```python
from build123d import *

# Parameters (mm, degrees)
BOSS_EXTRUDE1_DEPTH = 3.175
SHELL1_START        = -3.175
SHELL1_DEPTH        = 3.175
FILLET1_R           = 10.16
BOSS_EXTRUDE2_DEPTH = 3.175
SKETCH1_R           = 2.75
CUT_EXTRUDE1_DEPTH  = 81.407776093
EXTRUDE_THIN1_START = 25.4
SKETCH5_R           = 4.782
SKETCH5_R_2         = 2.75
EXTRUDE_THIN1_DEPTH = 25.4
SKETCH6_R           = 2.749999961
CUT_EXTRUDE2_DEPTH  = 85.264404295


# Read off the part's stored shape, not the designer's step: Shell1
with BuildPart() as part:
    # Sketch2 → Boss-Extrude1 (new body)
    with BuildSketch(Plane(origin=(0, 0, 0), x_dir=(1, 0, 0), z_dir=(0, 1, 0))):
        with BuildLine():
            Line((-60.494192364, -19.59062768), (-46.524192364, 43.90937232))
            ThreePointArc((-46.524192364, 43.90937232), (-42.81709678, 48.384476595), (-37.020836887, 47.969160828))
            Line((-37.020836887, 47.969160828), (50.609163113, -5.370839172))
            ThreePointArc((50.609163113, -5.370839172), (53.499476113, -12.202811), (47.939348616, -17.113486158))
            Line((47.939348616, -17.113486158), (-53.660651384, -27.273486158))
            ThreePointArc((-53.660651384, -27.273486158), (-59.037220059, -25.175205156), (-60.494192364, -19.59062768))
        make_face()
    extrude(amount=-BOSS_EXTRUDE1_DEPTH)

    # Shell1 outline → Shell1 (cut)
    with BuildSketch(Plane(origin=(0, 0, 0), x_dir=(1, 0, 0), z_dir=(0, 1, 0)).offset(SHELL1_START)):
        Polygon((-54.2925, -20.955), (47.3075, -10.795), (-40.3225, 42.545), align=None)
    extrude(amount=SHELL1_DEPTH, mode=Mode.SUBTRACT)

    # Fillet1
    fillet1_edges = [part.edges().sort_by_distance(p)[0] for p in [
        (-40.3225, -1.5875, -42.545),
        (47.3075, -1.5875, 10.795),
        (-54.2925, -1.5875, 20.955),
    ]]
    fillet(fillet1_edges, radius=FILLET1_R)

    # Sketch3 → Boss-Extrude2 (add)
    with BuildSketch(Plane(origin=(0, 0, 0), x_dir=(1, 0, 0), z_dir=(0, 1, 0))):
        with BuildLine():
            Line((-60.6425, -20.955), (-60.6425, -52.705))
            Line((-60.6425, -52.705), (53.6575, -52.705))
            Line((53.6575, -52.705), (53.6575, -10.795))
            ThreePointArc((53.6575, -10.795), (52.015723588, -15.055883787), (47.939348616, -17.113486158))
            Line((47.939348616, -17.113486158), (-53.660651384, -27.273486158))
            ThreePointArc((-53.660651384, -27.273486158), (-58.553383787, -25.663223588), (-60.6425, -20.955))
        make_face()
    extrude(amount=-BOSS_EXTRUDE2_DEPTH)

    # Sketch1 → Cut-Extrude1 (cut, through all)
    with BuildSketch(Plane(origin=(0, 0, 0), x_dir=(1, 0, 0), z_dir=(0, 1, 0))):
        with Locations(Location((-54.2925, -20.955, 0), (0, 0, 270))):
            Circle(SKETCH1_R)
        with Locations(Location((47.3075, -10.795, 0), (0, 0, 270))):
            Circle(SKETCH1_R)
        with Locations(Location((-40.3225, 42.545, 0), (0, 0, 270))):
            Circle(SKETCH1_R)
    extrude(amount=-CUT_EXTRUDE1_DEPTH, mode=Mode.SUBTRACT)

    # Sketch5 → Extrude-Thin1 (add)
    # profile 1 of 3: a face of its own
    with BuildSketch(Plane(origin=(0, 0, 0), x_dir=(1, 0, 0), z_dir=(0, 1, 0)).offset(EXTRUDE_THIN1_START)):
        with Locations((47.3075, -10.795)):
            Circle(SKETCH5_R)
        with Locations((47.3075, -10.795)):
            Circle(SKETCH5_R_2, mode=Mode.SUBTRACT)
    # profile 2 of 3: a face of its own
    with BuildSketch(Plane(origin=(0, 0, 0), x_dir=(1, 0, 0), z_dir=(0, 1, 0)).offset(EXTRUDE_THIN1_START)):
        with Locations((-54.2925, -20.955)):
            Circle(SKETCH5_R)
        with Locations((-54.2925, -20.955)):
            Circle(SKETCH5_R_2, mode=Mode.SUBTRACT)
    # profile 3 of 3: a face of its own
    with BuildSketch(Plane(origin=(0, 0, 0), x_dir=(1, 0, 0), z_dir=(0, 1, 0)).offset(EXTRUDE_THIN1_START)):
        with Locations((-40.3225, 42.545)):
            Circle(SKETCH5_R)
        with Locations((-40.3225, 42.545)):
            Circle(SKETCH5_R_2, mode=Mode.SUBTRACT)
    extrude(amount=-EXTRUDE_THIN1_DEPTH)

    # Sketch6 → Cut-Extrude2 (cut, through all)
    with BuildSketch(Plane(origin=(0, 0, 0), x_dir=(1, 0, 0), z_dir=(0, 1, 0))):
        with Locations(Location((-13.492499939, -42.705, 0), (0, 0, 270))):
            Circle(SKETCH6_R)
        with Locations(Location((6.507499939, -42.705, 0), (0, 0, 270))):
            Circle(SKETCH6_R)
    extrude(amount=-CUT_EXTRUDE2_DEPTH, mode=Mode.SUBTRACT)


solid = part.part
```
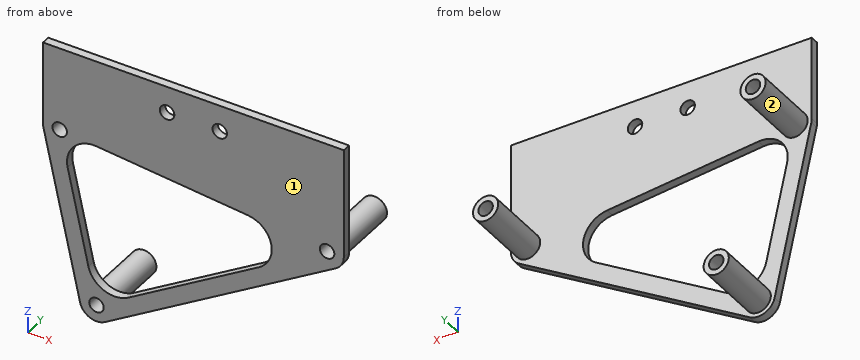
CAD build for the part. Positions are in the model's coordinates, mm. Face numbers are marked on the shaded views. A direction names the side the tool comes from. Give positions to 0.01 mm unless a question says otherwise; leave off trailing zeros. Write each loop counter-clockwise with the first axis right and the second up, starting at its lowest first coordinate (ties: lowest second). Pieces come first, ordered by that corner, then holes. Notation, with made-up numbers: M 80.25,9.25 L 99.25,9.25 A12 ccw 99.25,25.25 Z; hole C 29,52 d7. An arc over 180 degrees is marked long. Return JSON: item names as keys, results as strings. Group by question number.
(1) Drill centre lines: L1, parallel to Y at x = 45, z = 36.5 (3 decimals); L2, parallel to X at y = 5.75, z = 20; L3, parallel to Z at x = -41, y = 4.5. Where is each one in solid material? Low to high. Write a range as [from, to].
(2) Band-saw the part on B-B (y = 8.5). State how many separate pieces and enclosed holes the cut face has, and give its area (3 significant figures).
(3) Band-saw the part on A-A (x = 14). Give the cut face in (y, z) (3 decimals), and give its area (3 significant figures).
(4) 3-axis set-ups, long thin cutter, end or side, ignore diameter. For the marked faces 1 and 2: which of +Z, -Z, +X, -X, +Y, -Y reach the whole face in a straight line?
(5) Band-saw the part on D-D (z = 34). Give the cut face in (x, y) (1 decimal).
(6) Band-saw the part on C-C (z = -25.5). Give the cut face in (x, y) (3 decimals), and give its area (3 significant figures).
(7) Flat gauge pins, fed straight in: pin 1 Ø7 at (x, z) = (-13.49, 42.7) entering from -Y (3 decimals); pin 2 Ø6 at (x, y) = (-35.5, 6.5) entering from -Z; pin 3 Ø5 at (x, z) = (-54.29, 20.96) entering from -Y; pin 4 Ø7 at (x, z) = (6.51, 42.7) entering from +Y. Where does each tip first touch, or does it go through?
Entries:
{
 "1": {"L1": "y = [-3.175, 0]", "L2": "x = [-58.98, -56.87], [-51.71, -49.61]", "L3": "z = [-47.28, -45.21], [-39.88, -37.81]"},
 "2": {"separate pieces": "3", "enclosed holes": "3", "area": "144 mm^2"},
 "3": {"outline": "M -3.175,-16.913 L 0,-16.913 L 0,-9.479 L -3.175,-9.479 Z; M -3.175,14.126 L 0,14.126 L 0,52.705 L -3.175,52.705 Z", "area": "146 mm^2"},
 "4": {"face 1": "+Z, -Z, +X, -X, -Y", "face 2": "+Y"},
 "5": {"outline": "M -60.6,-3.2 L 53.7,-3.2 L 53.7,0 L -60.6,0 Z"},
 "6": {"outline": "M -50.574,-3.175 L -44.072,-3.175 L -44.072,0 L -50.574,0 Z; M -12.32,-3.175 L -0.107,-3.175 L -0.107,0 L -12.32,0 Z", "area": "59.4 mm^2"},
 "7": {"pin 1": "stops at y = -3.175", "pin 2": "stops at z = -46.97", "pin 3": "passes through", "pin 4": "stops at y = 0"}
}
